```python
from build123d import *

# Parameters (mm, degrees)
CUT_EXTRUDE1_DEPTH = 3.581396898


with BuildPart() as part:
    # Sketch2 → Base-Revolve (revolve)
    with BuildSketch(Plane.XY, mode=Mode.PRIVATE) as base_revolve_sk:
        Polygon((0, 0), (7.9375, 0), (7.9375, 6.35), (6.35, 7.9375), (0, 7.9375), align=None)
    revolve(base_revolve_sk.sketch.rotate(Axis((0, 0, 0), (0, 1, 0)), 90), axis=Axis((0, 0, 0), (0, 1, 0)))

    # Sketch3 → Boss-Revolve1 (revolve)
    with BuildSketch(Plane.XY, mode=Mode.PRIVATE) as boss_revolve1_sk:
        Polygon((0, -28.575), (3.96875, -28.575), (3.96875, -19.05), (3.175, -19.05), (3.175, -15.875), (4.7625, -15.875), (4.7625, -2.362197954), (4.445, -2.362197954), (4.445, 0), (0, 0), align=None)
    revolve(boss_revolve1_sk.sketch.rotate(Axis((0, 0, 0), (0, 1, 0)), 90), axis=Axis((0, 0, 0), (0, 1, 0)))

    # Sketch4 → Cut-Extrude1 (cut)
    with BuildSketch(Plane(origin=(0, 7.9375, 0), x_dir=(-1, 0, 0), z_dir=(0, 1, 0))):
        Polygon((2.387597932, 1.378480068), (6.25e-07, 2.756960497), (-2.387597307, 1.378481151), (-2.387598557, -1.378478985), (-1.876e-06, -2.756960497), (2.387596681, -1.378482234), align=None)
    extrude(amount=-CUT_EXTRUDE1_DEPTH, mode=Mode.SUBTRACT)


solid = part.part
```
Could you check a few things on this model? Use its own coordinates, in mm. A direction names the side the tool comes from. Give positions to 0.01 mm unless a question says otherwise; leave off trailing zeros. Loops run counter-clockwise (first coordinate to the right, second up) from the corner with the lowest first, then second, coordinate; pieces in that order, holes last. Notation, with made-up numbers: (-35.5, -38.5) -> (-1.5, -38.5) arc R7 cw to (-1.5, -26.5) -> close; hole circle Ø4 at (1.5, 89.25). An arc over 180 degrees is marked (long way). Put each result on its own line as item: value.
(1) Please list where these lines run through material, in increasing order: probe 1 along Y at (x, z) = (4.5, 0.75) (1 decimal); probe 2 along Y at (x, z) = (5, 0.75); probe 3 along X at (y, z) = (-7.5, 0). Write a range as [from, to].
Computed:
probe 1: [-15.9, -2.4], [0, 7.9]
probe 2: [0, 7.94]
probe 3: [-4.76, 4.76]
(2) Imagine slicing it at B-B on y = -7. Write out the boundary of the cut face in (x, z) (1 decimal), plus the area to 3 significant figures.
Computed:
outline: circle Ø9.5 at (0, 0)
area: 71.3 mm^2
(3) I'm going to push flat-ended pins straight in: pin 1 Ø4 at (x, y) = (-2, -3) entering from -Z; pin 2 Ø1 at (x, z) = (-1.5, -1.5) entering from +Y; pin 3 Ø6 at (x, y) = (4.5, -1) entering from +Z; pin 4 Ø2 at (x, y) = (4, -9.5) entering from +Z. Where does each tip first touch, or does it pass through?
Computed:
pin 1: z = -4.76
pin 2: y = 7.94
pin 3: z = 7.76
pin 4: z = 3.7
(4) For faces 4 (the face through (0, 7.938, -3)), 5 (the face through (-3, -19.05, 2)), 6 (the face through (0, 4.356, 0)), 7 (the face through (4.65, -9.02, 1.03)), which set-ups out of +Z, -Z, +X, -X, +Y, -Y let a thin tool reach every point of the face, with its end or its side?
Computed:
face 4: +Z, -Z, +X, -X, +Y
face 5: none
face 6: +Y
face 7: -Y
(5) Imagine slicing it at C-C on y = -20.5. Write out the boundary of the cut face in (x, z), plus the area to 3 significant figures.
Computed:
outline: circle Ø7.94 at (0, 0)
area: 49.5 mm^2
(6) Thinking about a two-plate mould opening in Z: for faces 1 (the face through (7.75, 3.22, 1.72)), 2 (the face through (3.4, 0, 3.4)), 3 (the face through (2.388, 6, 0)), which applies, pulls with the +Z half, pulls with the -Z half, needs draft (parallel to the pull), parting line crosses it, or undercut?
Computed:
face 1: parting line crosses it
face 2: needs draft
face 3: undercut
